The model under review builds one solid part; all positions refer to its coordinate system, in mm. A direction names the side the tool comes from. Round coordinates to 2 decimals unless told otherwise and drop trailing zeros. Order: outer loops, then holes, each group sorted by start corner. A loop starts at its lowest first (then second) coordinate and runs counter-clockwise, first axis right, second up. Notation, with made-up numbers: M -14,-16 L 16,-16 A27 ccw 16,12 Z; hole C -13.75,14.5 d6. An arc over 180 degrees is marked long. Use a Markdown table: item, result. Add a question column.
1. Consider section C-C on z = 5.5. State the section outline as (x, y) points.
2. To check wall thickness, follow probe 1 along X at (y, z) = (25, 6.05); probe 2 along X at (y, z) = (41, 1.25); probe 3 along Z at (x, y) = (16, 14.5). State the ranges of each line that lie inside material, in increasing order.
3. For faces 1 (the flat face through (4, 25, 2)), 2 (the flat face through (24, 25, 8)), list the 3-axis set-ups (+Z, -Z, +X, -X, +Y, -Y) from which the entire face can be reached by the end or side of a thin tool; tool diameter is ignored.
4. The part is to be moulded in two halves that separate along Y. For faces 3 (the cylindrical face through (18.4, 26.2, 6)), 4 (the flat face through (20, 2, 4)), 5 (the flat face through (37, 25, 0)), 6 (the flat face through (16, 25, 4)), say which applies: +Y half, -Y half, draft (parallel to the pull), parting line (faces both ways), or undercut.
5. Consider section D-D on y = 37.5. State the section outline as (x, z) points.
6. Insertion check: P1, Ø3, axis at x = 17, z = 4, coming from the +Y side; P2, Ø1, axis at x = 10.5, y = 13, coming from the -Z side; P3, Ø3.5, axis at x = 20, y = 25, coming from the +Z side; P4, Ø4, axis at x = 31, z = 6.5, coming from the -Y side. Each pin has a flat end and moves straight along its axis. Give the tip position at first contact, or say it passes through.
7. Consider section A-A on x = 20. State the section outline as (y, z) points.
8. Consider section B-B on y = 25. State the section outline as (x, z) points.
from build123d import *

# Parameters (mm, degrees)
F1_DEPTH = 40
F2_R     = 0.5
F3_T     = 4
F4_R     = 2
F5_DEPTH = 4


# Not quite as in the source:
# - a shell that OpenCascade refuses in one call is made with other operations: the cavity is built on its own and cut out


with BuildPart() as f1:
    # F0 (on Right) → F1 (new body)
    with BuildSketch(Plane.YZ):
        Polygon((4, 8), (0, 0), (50, 0), (46, 8), align=None)
    extrude(amount=F1_DEPTH)

    # F2
    f2_edges = [f1.edges().sort_by_distance(p)[0] for p in [
        (20, 4, 8),
        (20, 46, 8),
        (20, 0, 0),
        (20, 50, 0),
    ]]
    fillet(f2_edges, radius=F2_R)

    # F3: shell of thickness 4, made by hand


with BuildPart() as f3_core1:
    # F3_t2: copy of F1
    add(f1.part)

    # the walls: a layer under each face that stays
    f3_faces = [f3_core1.faces().sort_by_distance(p)[0] for p in [
        (20, 2.1118033989, 4.2236067977),
        (0, 25, 4),
        (40, 25, 4),
        (20, 25, 8),
        (20, 47.8881966011, 4.2236067977),
    ]]
    thicken(f3_faces, amount=-F3_T, mode=Mode.SUBTRACT)


with BuildPart() as f1_1:
    add(f1.part)

    # what is left inside the walls is the cavity
    f3_cavity = [f3_core1.part.solids().sort_by_distance(p)[0] for p in [
        (25.333333, 25, 0.04),
    ]]
    add(f3_cavity, mode=Mode.SUBTRACT)

    # F4 (on face) → F5 (cut, through all)
    with BuildSketch(Plane(origin=(0, 0, 4), x_dir=(1, 0, 0), z_dir=(0, 0, -1))):
        with Locations((20, -25)):
            Circle(F4_R)
    extrude(amount=-F5_DEPTH, mode=Mode.SUBTRACT)


solid = f1_1.part
Answer block:
| question | item | result |
|---|---|---|
| 1 | outline | M 0,2.75 L 40,2.75 L 40,47.25 L 0,47.25 Z; hole C 20,25 d4 |
| 2 | probe 1 | 0 to 18, 22 to 40 |
| 2 | probe 2 | 0 to 4, 36 to 40 |
| 2 | probe 3 | 4 to 8 |
| 3 | face 1 | -Z |
| 3 | face 2 | +Z, +X, -X, +Y, -Y |
| 4 | face 3 | undercut |
| 4 | face 4 | -Y half |
| 4 | face 5 | draft |
| 4 | face 6 | undercut |
| 5 | outline | M 0,0 L 4,0 L 4,4 L 36,4 L 36,0 L 40,0 L 40,8 L 0,8 Z |
| 6 | P1 | y = 48.75 |
| 6 | P2 | z = 4 |
| 6 | P3 | through |
| 6 | P4 | y = 2.25 |
| 7 | outline | M 0.36,0.72 A0.5 ccw 0.81,0 L 4.47,0 L 6.47,4 L 23,4 L 23,8 L 4.31,8 A0.5 ccw 3.86,7.72 Z; M 27,4 L 43.53,4 L 45.53,0 L 49.19,0 A0.5 ccw 49.64,0.72 L 46.14,7.72 A0.5 ccw 45.69,8 L 27,8 Z |
| 8 | outline | M 0,0 L 4,0 L 4,4 L 18,4 L 18,8 L 0,8 Z; M 22,4 L 36,4 L 36,0 L 40,0 L 40,8 L 22,8 Z |
